The drawing under review shows one solid part. Ordinate dimensions are in mm from its lowest x, y, z. A direction names the side the tool comes from. Give positions to 0.01 mm unless a question says otherwise; leave off trailing zeros. Order: outer loops, then holes, each group sorted by start corner. A loop starts at its lowest first (then second) coordinate and runs counter-clockwise, first axis right, second up. Notation, with made-up numbers: (87.5, 53) -> (95.5, 53) arc R14 cw to (95.5, 70) -> close; hole circle Ø5 at (-12, -38.75). An arc over 180 degrees is marked (long way). One line per item, written item: value.
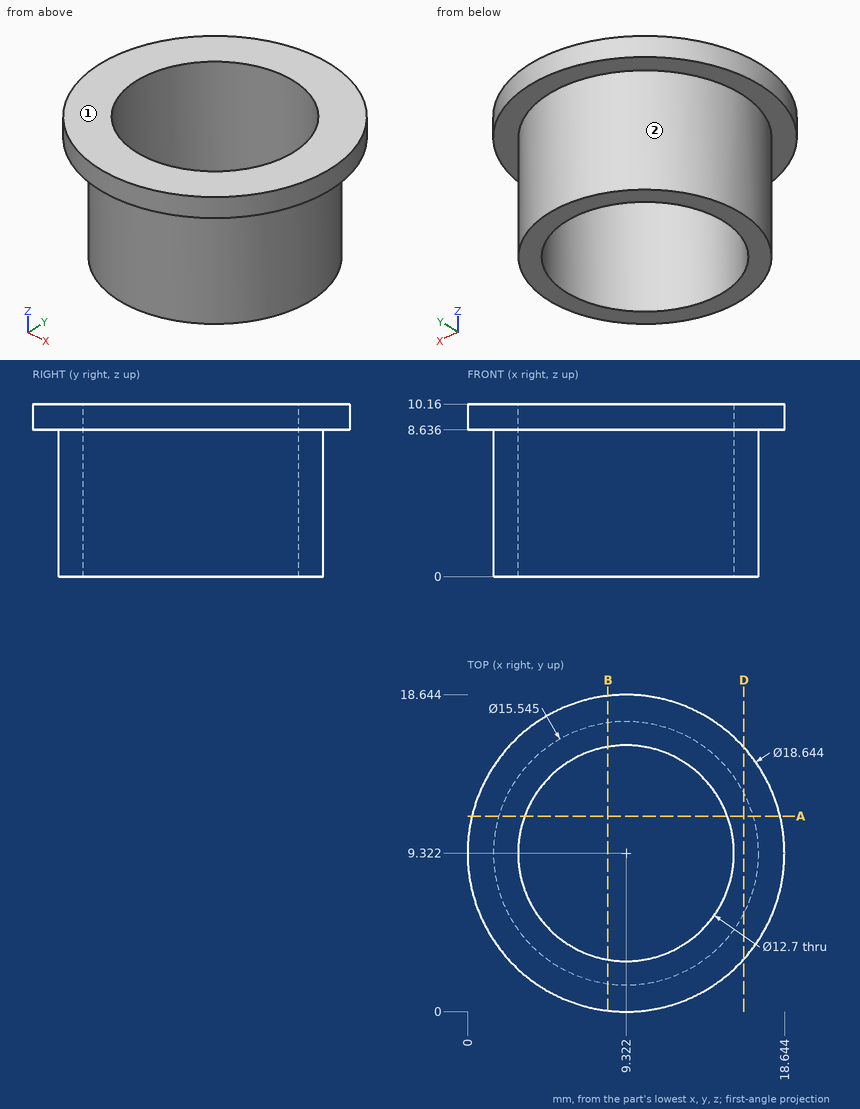
Item 1: Add section A-A on y = 11.5. Give the boundary of the cut face in (x, z) (1 decimal).
Returned:
outline: (0.3, 8.6) -> (1.9, 8.6) -> (1.9, 0) -> (3.4, 0) -> (3.4, 10.2) -> (0.3, 10.2) -> close; (15.3, 0) -> (16.8, 0) -> (16.8, 8.6) -> (18.4, 8.6) -> (18.4, 10.2) -> (15.3, 10.2) -> close
Item 2: To check wall thickness, follow line 1 along Z through (x, y) = (17.75, 7.75); line 2 along X through (y, z) = (4.25, 1.75) (1 decimal); line 3 along Y through (x, z) = (13, 5) (1 decimal). State the ranges of each line that lie inside material, in increasing order. Write a range as from..to.
Returned:
line 1: 8.64..10.16
line 2: 3.4..5.5, 13.1..15.2
line 3: 2.5..4.1, 14.5..16.2
Item 3: Clearance check with flat-ended pins moving along their axes: P1, Ø2, axis at y = 8.5, z = 1.5, coming from the +X side; P2, Ø1.5, axis at x = 11, z = 5.5, coming from the -Y side (1 decimal); P3, Ø4, axis at y = 13, z = 4, coming from the -X side. State where each tip first meets the part, or that it passes through.
Returned:
P1: x = 17.09
P2: y = 1.6
P3: x = 1.73
Item 4: Add section B-B on x = 8.25. Give the boundary of the cut face in (y, z), plus the area to 3 significant figures.
Returned:
outline: (0.06, 8.64) -> (1.62, 8.64) -> (1.62, 0) -> (3.06, 0) -> (3.06, 10.16) -> (0.06, 10.16) -> close; (15.58, 0) -> (17.02, 0) -> (17.02, 8.64) -> (18.58, 8.64) -> (18.58, 10.16) -> (15.58, 10.16) -> close
area: 34.0 mm²
Item 5: Add section D-D on x = 16.25. Give the boundary of the cut face in (y, z) (1 decimal).
Returned:
outline: (3.1, 8.6) -> (5.8, 8.6) -> (5.8, 0) -> (12.8, 0) -> (12.8, 8.6) -> (15.6, 8.6) -> (15.6, 10.2) -> (3.1, 10.2) -> close
Item 6: Machinability: for the marked faces 1 and 2, which of the approach directions +Z, -Z, +X, -X, +Y, -Y give a long, thin tool a straight path to every point of the face, cutting with its end or side? Answer none if there is none.
Returned:
face 1: +Z, +X, -X, +Y, -Y
face 2: -Z
